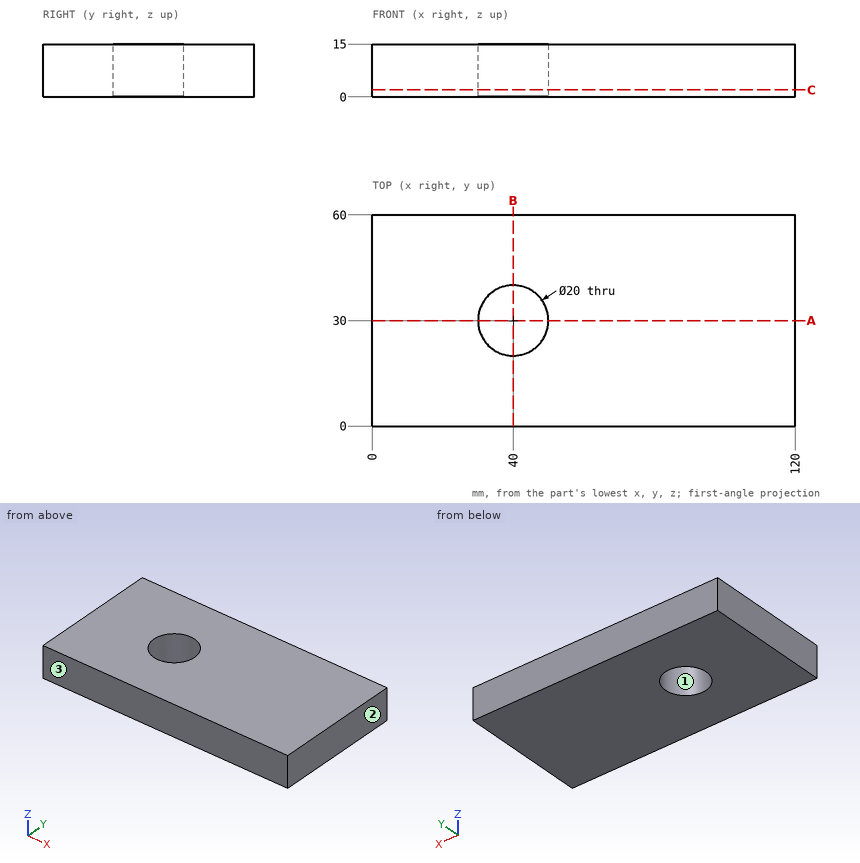
Source: three-view drawing plus pictorial views. Frame: mm from the lowest corner of the part. Round coordinates to 2 decimals unless told otherwise and drop trailing zeros. Order: outer loops, then holes, each group sorted by start corner. A loop starts at its lowest first (then second) coordinate and runs counter-clockwise, first axis right, second up. Notation, with made-up numbers: (-12, 69) - (1, 69) arc R33 cw to (1, 98) - close; hole circle Ø8 at (-19, -5). An arc over 180 degrees is marked (long way). Answer in a Markdown table with one row per item.
Item 1: Section query C-C (z = 2). Return the cut outline in (x, y), then the cut area to 3 significant figures.
Model answer:
| item | result |
|---|---|
| outline | (0, 0) - (120, 0) - (120, 60) - (0, 60) - close; hole circle Ø20 at (40, 30) |
| area | 6,890 mm² |
Item 2: Mould query, pull axis X, two halves, no side actions, for the marked faces 1, 2 and 3. Classes: released by +X, released by -X, zero draft, split by the parting line, or undercut.
Model answer:
| item | result |
|---|---|
| face 1 | undercut |
| face 2 | released by +X |
| face 3 | zero draft |
Item 3: Line query: line 1 (Y direction, x = 40, z = 10); line 2 (X direction, y = 22, z = 12); line 3 (X direction, y = 36.5, z = 9). Output: solid intervals per line, ascending.
Model answer:
| item | result |
|---|---|
| line 1 | y = 0 to 20, 40 to 60 |
| line 2 | x = 0 to 34, 46 to 120 |
| line 3 | x = 0 to 32.4, 47.6 to 120 |
Item 4: Pin query (flat end, axial travel): pin 1 (18 mm diameter, centred on x = 40, y = 30, fed in from +Z). Return the tip coordinate at first contact, or that it passes through.
Model answer:
| item | result |
|---|---|
| pin 1 | passes through |
Item 5: Section query B-B (x = 40). Return the cut outline in (y, z).
Model answer:
| item | result |
|---|---|
| outline | (0, 0) - (20, 0) - (20, 15) - (0, 15) - close; (40, 0) - (60, 0) - (60, 15) - (40, 15) - close |
Item 6: Section query A-A (y = 30). Return the cut outline in (x, z).
Model answer:
| item | result |
|---|---|
| outline | (0, 0) - (30, 0) - (30, 15) - (0, 15) - close; (50, 0) - (120, 0) - (120, 15) - (50, 15) - close |
